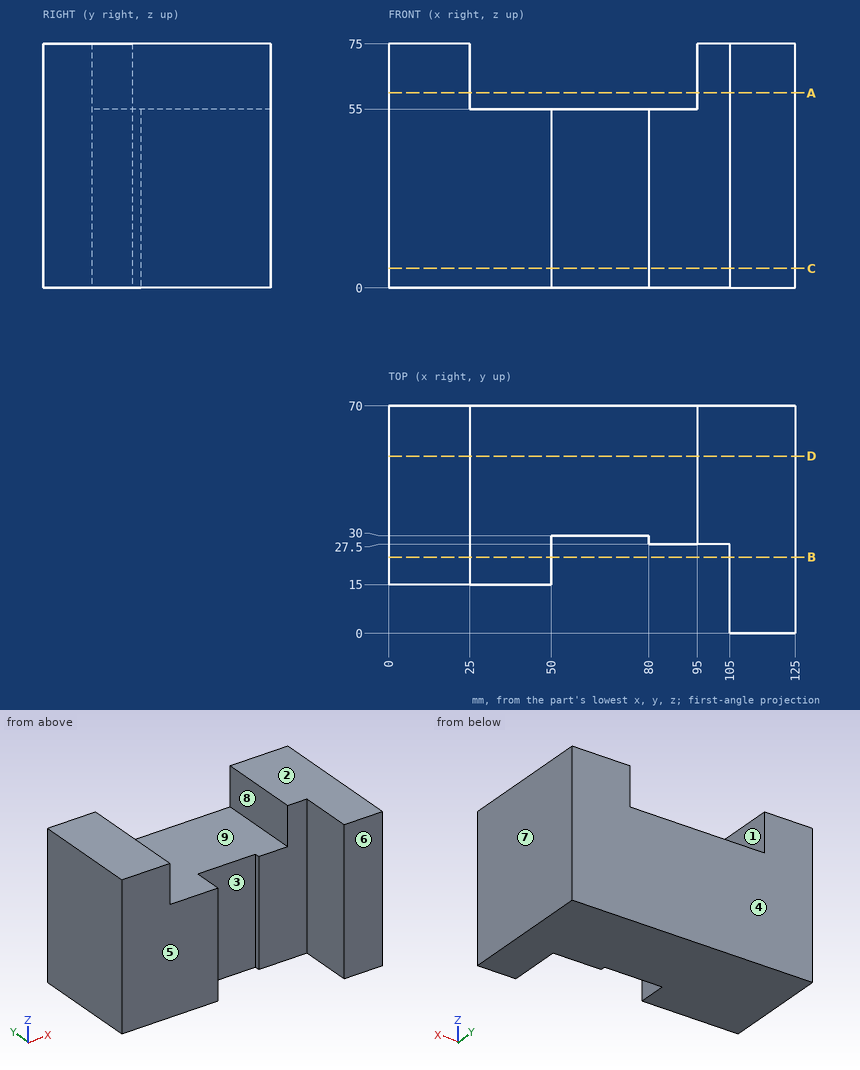
Can you work these out from the drawing? Everything is in mm from the part's minimum corner. A direction names the side the tool comes from. Coordinates: 2 decimals unless noted, no trailing zeros. Loops run counter-clockwise (first coordinate to the right, second up) from the corner with the lowest first, then second, coordinate; pieces in that order, holes last. Notation, with made-up numbers: (10.5, 88.25) - (69.5, 88.25) arc R21 ccw to (69.5, 117.25) - close; hole circle Ø5 at (-3, 9.25). An arc over 180 degrees is marked (long way). Use a Markdown table: item, result.
Item 1: Will these pins go through, and if not, where does the flat tip stop? pin 1 (12 mm diameter, centred on x = 62, z = 66, fed in from -Y); pin 2 (24 mm diameter, centred on x = 66, z = 31.5, fed in from -Y); pin 3 (12.5 mm diameter, centred on x = 90, z = 44, fed in from -Y); pin 4 (3 mm diameter, centred on x = 92, y = 55, fed in from +Z).
Numbers:
| item | result |
|---|---|
| pin 1 | passes through |
| pin 2 | stops at y = 30 |
| pin 3 | stops at y = 27.5 |
| pin 4 | stops at z = 55 |
Item 2: For the marked faces 1, 2, 3, 4 and 5, which set-ups out of +Z, -Z, +X, -X, +Y, -Y let a thin tool reach every point of the face, with its end or its side?
Numbers:
| item | result |
|---|---|
| face 1 | +Z, +Y, -Y |
| face 2 | +Z, +X, -X, +Y, -Y |
| face 3 | +Z, -Z, -Y |
| face 4 | +Z, -Z, +X, -X, +Y |
| face 5 | +Z, -Z, -X, -Y |
Item 3: I want a section at C-C on z = 6. Please give me the cut outline in (x, y).
Numbers:
| item | result |
|---|---|
| outline | (0, 15) - (50, 15) - (50, 30) - (80, 30) - (80, 27.5) - (105, 27.5) - (105, 0) - (125, 0) - (125, 70) - (0, 70) - close |
Item 4: I want a section at B-B on y = 23.5. Please give me the cut outline in (x, z).
Numbers:
| item | result |
|---|---|
| outline | (0, 0) - (50, 0) - (50, 55) - (25, 55) - (25, 75) - (0, 75) - close; (105, 0) - (125, 0) - (125, 75) - (105, 75) - close |
Item 5: I want a section at A-A on z = 60. Please give me the cut outline in (x, y).
Numbers:
| item | result |
|---|---|
| outline | (0, 15) - (25, 15) - (25, 70) - (0, 70) - close; (95, 27.5) - (105, 27.5) - (105, 0) - (125, 0) - (125, 70) - (95, 70) - close |
Item 6: We'd pull the mould along X, two halves only. Please class the marked faces 6, 7, 8 and 9: released by +X, released by -X, zero draft, split by the parting line, or undercut.
Numbers:
| item | result |
|---|---|
| face 6 | zero draft |
| face 7 | released by +X |
| face 8 | undercut |
| face 9 | undercut |
Item 7: I want a section at D-D on y = 54.5. Please give me the cut outline in (x, z), and give its area (4 significant figures).
Numbers:
| item | result |
|---|---|
| outline | (0, 0) - (125, 0) - (125, 75) - (95, 75) - (95, 55) - (25, 55) - (25, 75) - (0, 75) - close |
| area | 7,975 mm2 |
Item 8: If I drill on probe 1 along X at (y, z) = (36, 67.5); probe 2 along X at (y, z) = (24, 47); probe 3 along Y at (x, z) = (15.5, 35), over which ranges is the centre line in solid material (lowest first)? Write a range as from..to.
Numbers:
| item | result |
|---|---|
| probe 1 | x = 0..25, 95..125 |
| probe 2 | x = 0..50, 105..125 |
| probe 3 | y = 15..70 |
